The model under review builds one solid part; all positions refer to its coordinate system, in mm. Face numbers are marked on the shaded views. A direction names the side the tool comes from. Coordinates: 2 decimals unless noted, no trailing zeros. Write each loop counter-clockwise with the first axis right and the second up, starting at its lowest first coordinate (ties: lowest second). Pieces come first, ordered by that corner, then holes.
1) Add section B-B, the plane y = 20. State the section outline as (x, z) points.
2) For P1, Ø1.5, axis at x = -4.5, z = 10.5, coming from the +Y side; P2, Ø8, axis at y = 17, z = 20, coming from the -X side; P3, Ø5, axis at y = 5, z = 5, coming from the -X side, all flat-tipped, find the tip position at first contact; note any pin that passes through.
3) For line 1 (X direction, y = 25.5, z = 11.75); line 2 (X direction, y = 23.5, z = 9.5); line 3 (X direction, y = 5.75, z = 2), list the stretches that pass through material, from the lowest coordinate up.
4) Add section C-C, the plane x = -4. State the section outline as (y, z) points, then the cut area to 3 significant figures.
5) Machinability: for the marked faces 1 and 2, which of the approach directions +Z, -Z, +X, -X, +Y, -Y give a long, thin tool a straight path to every point of the face, cutting with its end or side? Answer none if there is none.
6) Add section A-A, the plane z = 9.5. State the section outline as (x, y) points.
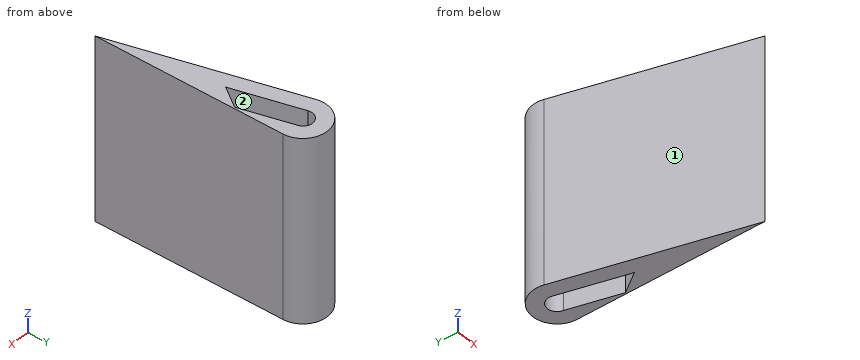
from build123d import *

# Parameters (mm, degrees)
F1_DEPTH = 25.4


with BuildPart() as f1:
    # F0 (on Top) → F1 (new body)
    with BuildSketch(Plane.XY):
        with BuildLine():
            Line((-6.574004, 24.534516), (0, 0))
            Line((0, 0), (0, 25.4))
            ThreePointArc((0, 25.4), (-3.78045, 28.715365), (-6.574004, 24.534516))
        make_face()
        with BuildLine():
            ThreePointArc((-4.620697, 25.097922), (-3.594908, 26.687752), (-2.04724, 25.599392))
            Line((-2.04724, 25.599392), (-0.198302, 18.69906))
            Line((-0.198302, 18.69906), (-2.155446, 15.897478))
            Line((-2.155446, 15.897478), (-4.600688, 25.023246))
            ThreePointArc((-4.600688, 25.023246), (-4.611242, 25.060436), (-4.620697, 25.097922))
        make_face(mode=Mode.SUBTRACT)
    extrude(amount=F1_DEPTH)


solid = f1.part
Geometry results:
1. outline: (-5.36, 0) - (-3.25, 0) - (-3.25, 25.4) - (-5.36, 25.4) - close; (-0.55, 0) - (0, 0) - (0, 25.4) - (-0.55, 25.4) - close
2. P1: stops at y = 28.72
2. P2: stops at x = -5.63
2. P3: stops at x = -2.01
3. line 1: x = -6.69 to -4.65, -2.02 to 0
3. line 2: x = -6.3 to -4.19, -1.48 to 0
3. line 3: x = -1.54 to 0
4. outline: (14.93, 0) - (22.78, 0) - (22.78, 25.4) - (14.93, 25.4) - close; (26.54, 0) - (28.68, 0) - (28.68, 25.4) - (26.54, 25.4) - close
4. area: 254 mm2
5. face 1: +Z, -Z, -X, -Y
5. face 2: +Z, -Z
6. outline: (-6.57, 24.53) - (0, 0) - (0, 25.4) arc R3.34 ccw (long way) to start; hole (-4.62, 25.1) arc R1.31 ccw to (-4.6, 25.02) - (-2.16, 15.9) - (-0.2, 18.7) - (-2.05, 25.6) arc R1.31 ccw (long way) to start
